Read the model definition and answer for the solid it produces. Units are mm, in the model's axes. A direction names the side the tool comes from. Give positions to 0.01 mm unless a question says otherwise; leave off trailing zeros. Answer as CSV lines item,"result".
```python
from build123d import *

# Parameters (mm, degrees)
SKETCH1_W           = 293
SKETCH1_H           = 75.5
BOSS_EXTRUDE1_DEPTH = 4.5
CUT_EXTRUDE1_REACH  = 153.352
SKETCH2_R           = 1.5


with BuildPart() as part:
    # Sketch1 → Boss-Extrude1 (new body)
    with BuildSketch(Plane.XY):
        Rectangle(SKETCH1_W, SKETCH1_H)
    extrude(amount=BOSS_EXTRUDE1_DEPTH)

    # Sketch2 → Cut-Extrude1 (cut, up to next)
    with BuildSketch(Plane.XY.offset(4.5), mode=Mode.PRIVATE) as cut_extrude1_sk1:
        with Locations((137, 28.25)):
            Circle(SKETCH2_R)
    cut_extrude1_tool1 = extrude(cut_extrude1_sk1.sketch, amount=-CUT_EXTRUDE1_REACH, mode=Mode.PRIVATE) & part.part
    # Sketch2 → Cut-Extrude1 (cut, up to next)
    with BuildSketch(Plane.XY.offset(4.5), mode=Mode.PRIVATE) as cut_extrude1_sk2:
        with Locations((-137, 28.25)):
            Circle(SKETCH2_R)
    cut_extrude1_tool2 = extrude(cut_extrude1_sk2.sketch, amount=-CUT_EXTRUDE1_REACH, mode=Mode.PRIVATE) & part.part
    # Sketch2 → Cut-Extrude1 (cut, up to next)
    with BuildSketch(Plane.XY.offset(4.5), mode=Mode.PRIVATE) as cut_extrude1_sk3:
        with Locations((-137, -32.75)):
            Circle(SKETCH2_R)
    cut_extrude1_tool3 = extrude(cut_extrude1_sk3.sketch, amount=-CUT_EXTRUDE1_REACH, mode=Mode.PRIVATE) & part.part
    # Sketch2 → Cut-Extrude1 (cut, up to next)
    with BuildSketch(Plane.XY.offset(4.5), mode=Mode.PRIVATE) as cut_extrude1_sk4:
        with Locations((137, -32.75)):
            Circle(SKETCH2_R)
    cut_extrude1_tool4 = extrude(cut_extrude1_sk4.sketch, amount=-CUT_EXTRUDE1_REACH, mode=Mode.PRIVATE) & part.part
    # Sketch2 → Cut-Extrude1 (cut, up to next)
    with BuildSketch(Plane.XY.offset(4.5), mode=Mode.PRIVATE) as cut_extrude1_sk5:
        with BuildLine():
            Line((2.5, -42.449938401), (-2.5, -42.449938401))
            ThreePointArc((-2.5, -42.449938401), (-7.199938401, -37.75), (-2.5, -33.050061599))
            Line((-2.5, -33.050061599), (2.5, -33.050061599))
            ThreePointArc((2.5, -33.050061599), (7.199938401, -37.75), (2.5, -42.449938401))
        make_face()
    cut_extrude1_tool5 = extrude(cut_extrude1_sk5.sketch, amount=-CUT_EXTRUDE1_REACH, mode=Mode.PRIVATE) & part.part
    add(cut_extrude1_tool1.solids().sort_by_distance((137, 28.25, 4.5))[0], mode=Mode.SUBTRACT)
    add(cut_extrude1_tool2.solids().sort_by_distance((-137, 28.25, 4.5))[0], mode=Mode.SUBTRACT)
    add(cut_extrude1_tool3.solids().sort_by_distance((-137, -32.75, 4.5))[0], mode=Mode.SUBTRACT)
    add(cut_extrude1_tool4.solids().sort_by_distance((137, -32.75, 4.5))[0], mode=Mode.SUBTRACT)
    add(cut_extrude1_tool5.solids().sort_by_distance((0, -37.75, 4.5))[0], mode=Mode.SUBTRACT)


solid = part.part
```
(1) For faces 1 (the cylindrical face through (-5.86, -34.463, 2.282)), 2 (the flat face through (-2, 1, 4.5)), determine the directions among +Z, -Z, +X, -X, +Y, -Y from which every point of the face is accessible in a straight line to the end or side of a thin tool.
Worked out:
face 1,"+Z, -Z, -Y"
face 2,"+Z, +X, -X, +Y, -Y"
(2) The mould has two halves that part along X. Classify faces 3 (the cylindrical face through (5.787, -34.39, 2.282)), 4 (the flat face through (-2, 1, 0)): +X half, -X half, draft (parallel to the pull), parting line (faces both ways), or undercut.
Worked out:
face 3,"undercut"
face 4,"draft"
(3) Find the intervals of material crossed by L1, parallel to Y at x = -137, z = 2.35; L2, parallel to X at y = 29, z = 4.2, in increasing order.
Worked out:
L1,"y = -37.75 to -34.25, -31.25 to 26.75, 29.75 to 37.75"
L2,"x = -146.5 to -138.3, -135.7 to 135.7, 138.3 to 146.5"
(4) Each of these flat-tipped pins is pushed along its axis until it touches: P1, Ø2.5, axis at x = -137, y = 28.25, coming from the +Z side; P2, Ø10, axis at x = -55.5, y = 10.5, coming from the -Z side. Where does it stop, or does it pass through?
Worked out:
P1,"passes through"
P2,"stops at z = 0"
